Geometry check sheet. Reference: the model listing, model coordinates, mm. Give positions to 0.01 mm unless a question says otherwise; leave off trailing zeros. Order: outer loops, then holes, each group sorted by start corner. A loop starts at its lowest first (then second) coordinate and runs counter-clockwise, first axis right, second up. Notation, with made-up numbers: M 11.25,61.5 L 32.25,61.5 A32 cw 32.25,94.5 Z; hole C 25,75 d8. An arc over 180 degrees is marked long. Answer as CSV lines item,"result". Start each with the question number.
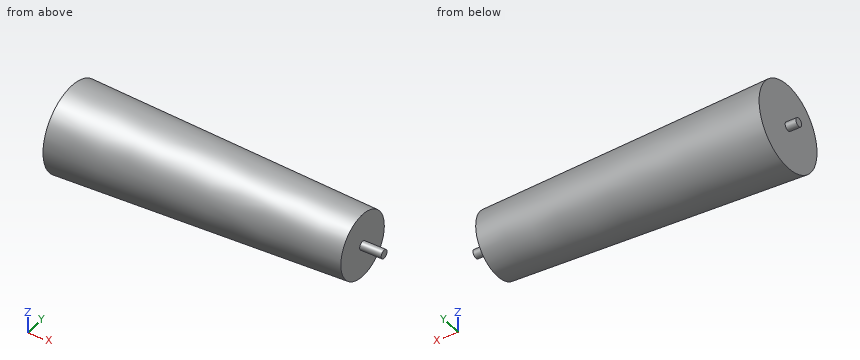
```python
from build123d import *

# Parameters (mm, degrees)
SKETCH1_R                = 40
SKETCH2_R                = 30
SKETCH3_R                = 4
BOSS_EXTRUDE1_DEPTH      = 20
BOSS_EXTRUDE1_DEPTH_BACK = 280


with BuildPart() as part:
    # Sketch1 → Loft1 section 0
    with BuildSketch(Plane(origin=(0, 0, 0), x_dir=(0, 0, -1), z_dir=(1, 0, 0))):
        Circle(SKETCH1_R)
    # Sketch2 → Loft1 section 1
    with BuildSketch(Plane(origin=(270, 0, 0), x_dir=(0, 0, -1), z_dir=(1, 0, 0))):
        Circle(SKETCH2_R)
    loft()

    # Sketch3 → Boss-Extrude1 (add, two sides)
    with BuildSketch(Plane(origin=(270, 0, 0), x_dir=(0, 0, -1), z_dir=(1, 0, 0))) as boss_extrude1_sk:
        Circle(SKETCH3_R)
    extrude(amount=BOSS_EXTRUDE1_DEPTH)
    extrude(boss_extrude1_sk.sketch, amount=-BOSS_EXTRUDE1_DEPTH_BACK)


solid = part.part
```
Item 1: Section check A-A on z = 0. Record the boundary of the cut face in (x, y).
Item 2: Scan lines: line 1 along X through (y, z) = (17, 13.5); line 2 along Z through (x, y) = (191, -6.5); line 3 along Y through (x, z) = (117, -18). Record each from-to range of solid material in increasing order.
Item 3: Depth check by flat-ended pin: pin 1 Ø3 at (y, z) = (-21.5, -29) entering from -X; pin 2 Ø5 at (x, y) = (155.5, 14) entering from -Z; pin 3 Ø2 at (x, y) = (194.5, 16) entering from +Z. Enter the tip coordinate at first touch or a pass-through.
Item 4: Section check B-B on x = 148.5. Record the boundary of the cut face in (y, z), then the cut area to 3 significant figures.
Item 5: Section check C-C on x = 253.5. Record the boundary of the cut face in (y, z), then the cut area to 3 significant figures.
Numbers:
1,outline,"M -10,-4 L 0,-4 L 0,-40 L 270,-30 L 270,-4 L 290,-4 L 290,4 L 270,4 L 270,30 L 0,40 L 0,4 L -10,4 Z"
2,line 1,"0 to 270"
2,line 2,"-32.28 to 32.28"
2,line 3,"-30.79 to 30.79"
3,pin 1,"x = 0"
3,pin 2,"z = -32.26"
3,pin 3,"z = 29.17"
4,outline,"C 0,0 d69"
4,area,"3,740 mm2"
5,outline,"C 0,0 d61.22"
5,area,"2,940 mm2"
